```python
from build123d import *

# Parameters (mm, degrees)
SKETCH_1_W          = 65
SKETCH_1_H          = 25
SKETCH_1_R          = 3.05
EXTRUDE_1_DEPTH     = 3
CUT_EXTRUDE_1_DEPTH = 4
SKETCH_3_W          = 65
SKETCH_3_H          = 3
EXTRUDE_2_DEPTH     = 50
SKETCH_4_R          = 1.6
SKETCH_4_R_2        = 6.1
CUT_EXTRUDE_4_DEPTH = 40
SKETCH_5_R          = 2.1
CUT_EXTRUDE_5_DEPTH = 10
SKETCH_6_R          = 2.1
CUT_EXTRUDE_6_DEPTH = 10


with BuildPart() as part:
    # ｽｹｯﾁ1 → ﾎﾞｽ - 押し出し1 (new body)
    with BuildSketch(Plane.XY):
        Rectangle(SKETCH_1_W, SKETCH_1_H)
        with Locations((-19.83, 7)):
            Circle(SKETCH_1_R, mode=Mode.SUBTRACT)
        with Locations((19.83, 7)):
            Circle(SKETCH_1_R, mode=Mode.SUBTRACT)
    extrude(amount=EXTRUDE_1_DEPTH)

    # ｽｹｯﾁ2 → ｶｯﾄ - 押し出し1 (cut, through all)
    with BuildSketch(Plane.XY.offset(3)):
        with BuildLine():
            ThreePointArc((-27.9, 7.5), (-28.36862915, 8.63137085), (-29.5, 9.1))
            Line((-29.5, 9.1), (-29.5, 7.5))
            Line((-29.5, 7.5), (-31.1, 7.5))
            ThreePointArc((-31.1, 7.5), (-29.5, 5.9), (-27.9, 7.5))
        make_face()
        with BuildLine():
            Line((-29.5, 7.5), (-29.5, 9.1))
            ThreePointArc((-29.5, 9.1), (-30.63137085, 8.63137085), (-31.1, 7.5))
            Line((-31.1, 7.5), (-29.5, 7.5))
        make_face()
        with BuildLine():
            ThreePointArc((-31.1, -7.5), (-30.63137085, -8.63137085), (-29.5, -9.1))
            Line((-29.5, -9.1), (-29.5, -7.5))
            Line((-29.5, -7.5), (-31.1, -7.5))
        make_face()
        with BuildLine():
            Line((-29.5, -7.5), (-29.5, -9.1))
            ThreePointArc((-29.5, -9.1), (-28.36862915, -8.63137085), (-27.9, -7.5))
            ThreePointArc((-27.9, -7.5), (-29.5, -5.9), (-31.1, -7.5))
            Line((-31.1, -7.5), (-29.5, -7.5))
        make_face()
        with BuildLine():
            ThreePointArc((31.1, 7.5), (30.63137085, 8.63137085), (29.5, 9.1))
            Line((29.5, 9.1), (29.5, 7.5))
            Line((29.5, 7.5), (31.1, 7.5))
        make_face()
        with BuildLine():
            Line((29.5, 7.5), (29.5, 9.1))
            ThreePointArc((29.5, 9.1), (28.36862915, 6.36862915), (31.1, 7.5))
            Line((31.1, 7.5), (29.5, 7.5))
        make_face()
        with BuildLine():
            ThreePointArc((31.1, -7.5), (28.36862915, -6.36862915), (29.5, -9.1))
            Line((29.5, -9.1), (29.5, -7.5))
            Line((29.5, -7.5), (31.1, -7.5))
        make_face()
        with BuildLine():
            Line((29.5, -7.5), (29.5, -9.1))
            ThreePointArc((29.5, -9.1), (30.63137085, -8.63137085), (31.1, -7.5))
            Line((31.1, -7.5), (29.5, -7.5))
        make_face()
    extrude(amount=-CUT_EXTRUDE_1_DEPTH, mode=Mode.SUBTRACT)

    # ｽｹｯﾁ3 → ﾎﾞｽ - 押し出し2 (add)
    with BuildSketch(Plane(origin=(0, 12.5, 0), x_dir=(1, 0, 0), z_dir=(0, 1, 0))):
        with Locations((0, -1.5)):
            Rectangle(SKETCH_3_W, SKETCH_3_H)
    extrude(amount=EXTRUDE_2_DEPTH)

    # ｽｹｯﾁ4 → ｶｯﾄ - 押し出し4 (cut)
    with BuildSketch(Plane.XY):
        with Locations((-7.875, 57.13990011)):
            Circle(SKETCH_4_R)
        with Locations((7.875, 57.13990011)):
            Circle(SKETCH_4_R)
        with Locations((15.75, 43.5)):
            Circle(SKETCH_4_R)
        with Locations((7.875, 29.86009989)):
            Circle(SKETCH_4_R)
        with Locations((-7.875, 29.86009989)):
            Circle(SKETCH_4_R)
        with Locations((-15.75, 43.5)):
            Circle(SKETCH_4_R)
        with Locations((0, 50.5)):
            Circle(SKETCH_4_R_2)
    extrude(amount=CUT_EXTRUDE_4_DEPTH, mode=Mode.SUBTRACT)

    # ｽｹｯﾁ5 → ｶｯﾄ - 押し出し5 (cut)
    with BuildSketch(Plane(origin=(0, 0, 0), x_dir=(-1, 0, 0), z_dir=(0, 0, -1))):
        with Locations((-26.360896025, 26)):
            Circle(SKETCH_5_R)
    extrude(amount=-CUT_EXTRUDE_5_DEPTH, mode=Mode.SUBTRACT)

    # ｽｹｯﾁ6 → ｶｯﾄ - 押し出し6 (cut)
    with BuildSketch(Plane.XY.offset(3)):
        with Locations((-26.36, 26)):
            Circle(SKETCH_6_R)
    extrude(amount=-CUT_EXTRUDE_6_DEPTH, mode=Mode.SUBTRACT)


solid = part.part
```
Here's how the part is built. I have some questions about the finished solid (model axes, mm). Round coordinates to 2 decimals unless told otherwise and drop trailing zeros. Write each loop counter-clockwise with the first axis right and the second up, starting at its lowest first coordinate (ties: lowest second). Pieces come first, ordered by that corner, then holes.
Q1. Please list where these lines run through material, in increasing order: probe 1 along X at (y, z) = (24.5, 0.4); probe 2 along X at (y, z) = (58, 0.25); probe 3 along Y at (x, z) = (-19.83, 0.9).
Q2. If we section it at A-A on x = -15.75: Write out the boundary of the cut face in (y, z).
Q3. If we mould it in two halves opening along Y, with no side actions, what happens to faces 1 (the flat face through (0, -12.5, 1)), 2 (the flat face through (-32.5, 24, 2)), 3 (the cylindrical face through (14.5, 42.5, 1.5))? For each: +Y half, -Y half, draft (parallel to the pull), parting line (faces both ways), or undercut.
Q4. If we section it at C-C on z = 2.4: Give the number of separate pieces and of enclosed holes in the cut face, plus the area to 3 significant figures.
Q5. If we section it at B-B on y = 50.5: Write out the boundary of the cut face in (x, z), plus the area to 3 significant figures.
Answer below:
1. probe 1: x = -32.5 to -27.83, -24.89 to 24.89, 27.83 to 32.5
1. probe 2: x = -32.5 to -9.22, -6.53 to 6.53, 9.22 to 32.5
1. probe 3: y = -12.5 to 3.95, 10.05 to 62.5
2. outline: (-12.5, 0) - (41.9, 0) - (41.9, 3) - (-12.5, 3) - close; (45.1, 0) - (62.5, 0) - (62.5, 3) - (45.1, 3) - close
3. face 1: -Y half
3. face 2: draft
3. face 3: undercut
4. separate pieces: 1
4. enclosed holes: 15
4. area: 4,590 mm2
5. outline: (-32.5, 0) - (-6.1, 0) - (-6.1, 3) - (-32.5, 3) - close; (6.1, 0) - (32.5, 0) - (32.5, 3) - (6.1, 3) - close
5. area: 158 mm2
